```python
from build123d import *

# Parameters (mm, degrees)
F0_R     = 29.2481
F1_DEPTH = 25.4
F2_SIZE  = 0.762
F4_D     = 5.1054


with BuildPart() as f1:
    # F0 (on Top) → F1 (new body)
    with BuildSketch(Plane.XY):
        Circle(F0_R)
    extrude(amount=F1_DEPTH)

    # F2
    f2_edges = [f1.edges().sort_by_distance(p)[0] for p in [
        (-29.2481, 0, 25.4),
        (-29.2481, 0, 0),
    ]]
    chamfer(f2_edges, length=F2_SIZE)

    # F4 (through all)
    with Locations(Plane.XY.offset(25.4)):
        with Locations((0, 0)):
            Hole(F4_D / 2)


solid = f1.part
```
CAD build for the part. Positions are in the model's coordinates, mm. Round coordinates to 2 decimals unless told otherwise and drop trailing zeros. Write each loop counter-clockwise with the first axis right and the second up, starting at its lowest first coordinate (ties: lowest second). Pieces come first, ordered by that corner, then holes. Notation, with made-up numbers: (63, 60.5) -> (93, 60.5) arc R34 ccw to (93, 91.5) -> close; hole circle Ø2 at (-2, 32). An arc over 180 degrees is marked (long way). Answer in a Markdown table with one row per item. Add a question column.
Item 1: Drop flat-ended pins along their axis: pin 1 Ø5 at (y, z) = (10, 13) entering from -X; pin 2 Ø1.5 at (x, y) = (-10, -16) entering from -Z; pin 3 Ø2 at (y, z) = (-5.5, 7) entering from +X; pin 4 Ø8 at (x, z) = (10.5, 15) entering from -Y. Give the stop position or say it passes through.
Item 2: Saw through at C-C, the plane z = 5.5. Write the cut outline in (x, y), then the cut area to 3 significant figures.
Item 3: Mould opens along Y. For faces 1 (the face through (-2.435, 0.767, 12.522)), 2 (the face through (0, -6, 25.4)), 3 (the face through (-6.34, -28.553, 12.533)) say: pulls with the +Y half, pulls with the -Y half, needs draft (parallel to the pull), parting line crosses it, or undercut.
Item 4: Saw through at A-A, the plane y = 0. Write the cut outline in (x, z).
Item 5: Drill centre lines: line 1 (Y direction, x = 0, z = 20); line 2 (Y direction, x = -2, z = 18.5); line 3 (Y direction, x = -23.5, z = 13.75). Where is each one in solid material? Low to high. Write a range as from..to.
Findings below:
| question | item | result |
|---|---|---|
| 1 | pin 1 | stops at x = -28.27 |
| 1 | pin 2 | stops at z = 0 |
| 1 | pin 3 | stops at x = 28.9 |
| 1 | pin 4 | stops at y = -28.52 |
| 2 | outline | circle Ø58.5 at (0, 0); hole circle Ø5.11 at (0, 0) |
| 2 | area | 2,670 mm^2 |
| 3 | face 1 | undercut |
| 3 | face 2 | needs draft |
| 3 | face 3 | parting line crosses it |
| 4 | outline | (-29.25, 0.76) -> (-28.49, 0) -> (-2.55, 0) -> (-2.55, 25.4) -> (-28.49, 25.4) -> (-29.25, 24.64) -> close; (2.55, 0) -> (28.49, 0) -> (29.25, 0.76) -> (29.25, 24.64) -> (28.49, 25.4) -> (2.55, 25.4) -> close |
| 5 | line 1 | y = -29.25..-2.55, 2.55..29.25 |
| 5 | line 2 | y = -29.18..-1.59, 1.59..29.18 |
| 5 | line 3 | y = -17.41..17.41 |
